CAD build for the part. Positions are in the model's coordinates, mm. Round coordinates to 2 decimals unless told otherwise and drop trailing zeros. Loops run counter-clockwise (first coordinate to the right, second up) from the corner with the lowest first, then second, coordinate; pieces in that order, holes last. Notation, with made-up numbers: (53.5, 36.5) - (67.5, 36.5) arc R13 ccw to (67.5, 59.5) - close; hole circle Ø11 at (83, 0). An arc over 180 degrees is marked (long way). One line per question, with ' | ' between items.
```python
from build123d import *

# Parameters (mm, degrees)
F1_DEPTH = 7.5
F2_SIZE  = 5
F5_R     = 4
F6_DEPTH = 15.001


# Not quite as in the source:
# - two fillets or chamfers of one size are made in one step


with BuildPart() as f1:
    # F0 (on Front) → F1 (new body, symmetric)
    with BuildSketch(Plane.XZ):
        with BuildLine():
            Line((110, 60), (110, 110))
            Line((110, 110), (50, 110))
            ThreePointArc((50, 110), (0, 60), (-50, 110))
            Line((-50, 110), (-110, 110))
            Line((-110, 110), (-110, 60))
            ThreePointArc((-110, 60), (-67.5735931288, 42.4264068712), (-50, 0))
            ThreePointArc((-50, 0), (-67.5735931288, -42.4264068712), (-110, -60))
            Line((-110, -60), (-110, -110))
            Line((-110, -110), (110, -110))
            Line((110, -110), (110, -60))
            ThreePointArc((110, -60), (50, 0), (110, 60))
        make_face()
    extrude(amount=F1_DEPTH, both=True)

    # F2
    f2_edges = [f1.edges().sort_by_distance(p)[0] for p in [
        (-110, 7.5, -85),
        (-110, 7.5, 85),
        (110, 7.5, 85),
        (110, 7.5, -85),
        (110, -7.5, 85),
        (110, -7.5, -85),
        (-110, -7.5, -85),
        (-110, -7.5, 85),
    ]]
    chamfer(f2_edges, length=F2_SIZE)

    # F5 (on face) → F6 (cut, through all)
    with BuildSketch(Plane.XZ.offset(7.5)):
        with Locations((0, 29.5)):
            Circle(F5_R)
    extrude(amount=-F6_DEPTH, mode=Mode.SUBTRACT)


solid = f1.part
```
(1) Probe L1, parallel to Z at x = 0, y = 0.75; L2, parallel to X at y = -0.5, z = 31.5; L3, parallel to Z at x = 95, y = -6. List the from-to ranges inside material, lowest first.
Results found:
L1: z = -110 to 25.5, 33.5 to 60 | L2: x = -58.93 to -3.46, 3.46 to 58.93 | L3: z = -110 to -58.09, 58.09 to 110
(2) Cut at B-B, the plane z = -65. Write the cut outline in (x, y), then the cut area to 3 significant figures.
Results found:
outline: (-110, -2.5) - (-105, -7.5) - (105, -7.5) - (110, -2.5) - (110, 2.5) - (105, 7.5) - (-105, 7.5) - (-110, 2.5) - close | area: 3,250 mm²
(3) Cut at C-C, the plane z = 92. Write the cut outline in (x, y).
Results found:
outline: (-110, -2.5) - (-105, -7.5) - (-46.65, -7.5) - (-46.65, 7.5) - (-105, 7.5) - (-110, 2.5) - close; (46.65, -7.5) - (105, -7.5) - (110, -2.5) - (110, 2.5) - (105, 7.5) - (46.65, 7.5) - close
(4) Two-plate mould, pull along X, no slides. Class faces 1 (the face through (107.5, -5, 84.5)), 2 (the face through (-0.521, -0.105, 33.466)), 3 (the face through (80, 0, 110)): released by +X, released by -X, zero draft, split by the parting line, or undercut.
Results found:
face 1: released by +X | face 2: undercut | face 3: zero draft
(5) Cut at D-D, the plane x = -60. Write the cut outline in (y, z).
Results found:
outline: (-7.5, -110) - (7.5, -110) - (7.5, -33.17) - (-7.5, -33.17) - close; (-7.5, 33.17) - (7.5, 33.17) - (7.5, 110) - (-7.5, 110) - close
(6) Drop flat-ended pins along their axis: P1, Ø5, axis at x = -23.5, y = 0, coming from the +Z side; P2, Ø8, axis at y = 5.5, z = 3.5, coming from the -X side; P3, Ø6, axis at y = -4, z = -19.5, coming from the -X side. Give the stop position or say it passes through.
Results found:
P1: stops at z = 67.29 | P2: stops at x = -50.47 | P3: stops at x = -54.38
(7) Cut at A-A, the plane x = 0. Write the cut outline in (y, z), then the cut area to 3 significant figures.
Results found:
outline: (-7.5, -110) - (7.5, -110) - (7.5, 25.5) - (-7.5, 25.5) - close; (-7.5, 33.5) - (7.5, 33.5) - (7.5, 60) - (-7.5, 60) - close | area: 2,430 mm²
